For this review, take the finished solid that the model builds, in its own axes (mm). A direction names the side the tool comes from. Round coordinates to 2 decimals unless told otherwise and drop trailing zeros. Write each loop counter-clockwise with the first axis right and the second up, starting at its lowest first coordinate (ties: lowest second). Pieces come first, ordered by that corner, then holes. Notation, with made-up numbers: (82, 74.25) -> (106, 74.25) arc R21 cw to (106, 108.25) -> close; hole circle Ø4 at (17.5, 23). An arc over 180 degrees is marked (long way). Answer as CSV lines item,"result". Start each with the question number.
Item 1: Take a section at B-B on z = 0. Give the boundary of the cut face in (x, y), then the cut area to 3 significant figures.
Item 2: For pin 1 Ø7.5 at (x, z) = (-30.17, 0) entering from +Y; pin 2 Ø4 at (x, y) = (-39.5, -19) entering from +Z; pin 3 Ø14 at (x, z) = (-30.17, 0) entering from -Y, all flat-tipped, find the tip position at first contact; note any pin that passes through.
Item 3: Take a section at A-A on y = -32.5. Give the boundary of the cut face in (x, z).
Item 4: Take a section at D-D on z = 45. Give the boundary of the cut face in (x, y), then the cut area to 3 significant figures.
Item 5: Machinability: for faces 1 (the flat face through (-12, -12, 50)), 2 (the flat face through (-1, -50, 3)), which of the approach directions +Z, -Z, +X, -X, +Y, -Y give a long, thin tool a straight path to every point of the face, cutting with its end or side? Answer none if there is none.
Item 6: Take a section at C-C on x = 35. Give the boundary of the cut face in (y, z).
Item 7: Mouldability with a two-part tool opening along Z and no side actions: class faces 3 (the cylindrical face through (-35.94, -14.12, 1.82)), 4 (the cylindrical face through (1, -48, -49)), 5 (the flat face through (16, 29, 75)) as +Z half, -Z half, draft (parallel to the pull), parting line (faces both ways), or undercut.
Item 8: Wall thickness on probe 1 along X at (y, z) = (3, 0); probe 2 along Z at (x, y) = (45.5, 15); probe 3 along Y at (x, z) = (-33.5, -7): over which ranges is each line inside the solid? List them lowest first. Write a range as from..to.
```python
from build123d import *

# Parameters (mm, degrees)
F0_W      = 100
F0_H      = 100
F1_DEPTH  = 50
F2_R      = 10
F3_DEPTH  = 105
F4_R      = 6.050318
F5_DEPTH  = 105
F6_R      = 5
F7_R      = 15.676311
F8_DEPTH  = 25
F10_DEPTH = 25


with BuildPart() as f1:
    # F0 (on Front) → F1 (new body, symmetric)
    with BuildSketch(Plane.XZ):
        Rectangle(F0_W, F0_H)
    extrude(amount=F1_DEPTH, both=True)

    # F2 (on face) → F3 (cut)
    with BuildSketch(Plane.XY.offset(50)):
        with Locations((-27.335882, 25.35297)):
            Circle(F2_R)
    extrude(amount=-F3_DEPTH, mode=Mode.SUBTRACT)

    # F4 (on face) → F5 (cut)
    with BuildSketch(Plane(origin=(0, 50, 0), x_dir=(-1, 0, 0), z_dir=(0, 1, 0))):
        with Locations((30.168613, 0)):
            Circle(F4_R)
    extrude(amount=-F5_DEPTH, mode=Mode.SUBTRACT)

    # F6
    f6_edges = [f1.edges().sort_by_distance(p)[0] for p in [
        (0, 50, -50),
        (-50, 0, -50),
        (50, 0, -50),
        (0, -50, -50),
        (-37.335882, 25.35297, -50),
    ]]
    fillet(f6_edges, radius=F6_R)

    # F7 (on face) → F8 (join)
    with BuildSketch(Plane.XY.offset(50)):
        Circle(F7_R)
    extrude(amount=F8_DEPTH)

    # F9 (on face) → F10 (join)
    with BuildSketch(Plane.XY.offset(50)):
        with BuildLine():
            add(Edge.make_bspline(
                [(4.390738, 34.417719), (-0.534371, 24.049071), (18.924589, 21.160099), (38.383548, 18.271128), (23.849698, 31.528747), (9.315848, 44.786366), (4.390738, 34.417719)],
                knots=[0, 0, 0, 2.094395, 2.094395, 4.18879, 4.18879, 6.283185, 6.283185, 6.283185], degree=2, weights=[1, 0.5, 1, 0.5, 1, 0.5, 1]))
        make_face()
    extrude(amount=F10_DEPTH)


solid = f1.part
```
Output values:
1,outline,"(-50, -50) -> (-36.22, -50) -> (-36.22, 20.76) arc R10 cw to (-36.22, 29.95) -> (-36.22, 50) -> (-50, 50) -> close; (-24.12, -50) -> (50, -50) -> (50, 50) -> (-24.12, 50) -> (-24.12, 34.82) arc R10 cw to (-24.12, 15.88) -> close"
1,area,"8,690 mm^2"
2,pin 1,"passes through"
2,pin 2,"stops at z = 50"
2,pin 3,"stops at y = -50"
3,outline,"(-50, -45) arc R5 ccw to (-45, -50) -> (45, -50) arc R5 ccw to (50, -45) -> (50, 50) -> (-50, 50) -> close; hole circle Ø12.1 at (-30.17, 0)"
4,outline,"(-50, -50) -> (50, -50) -> (50, 50) -> (-50, 50) -> close; hole circle Ø20 at (-27.34, 25.35)"
4,area,"9,690 mm^2"
5,face 1,"+Z"
5,face 2,"+Z, -Z, +X, -X, -Y"
6,outline,"(-50, -45) arc R5 ccw to (-45, -50) -> (45, -50) arc R5 ccw to (50, -45) -> (50, 50) -> (-50, 50) -> close"
7,face 3,"undercut"
7,face 4,"-Z half"
7,face 5,"+Z half"
8,probe 1,"x = -50..-36.22, -24.12..50"
8,probe 2,"z = -49.97..50"
8,probe 3,"y = -50..17.48, 33.23..50"
